Geometry: final body of the model. Coordinates: model frame, mm. Face numbers are marked on the shaded views. A direction names the side the tool comes from. Give positions to 0.01 mm unless a question says otherwise; leave off trailing zeros. Write each loop counter-clockwise with the first axis right and the second up, starting at its lowest first coordinate (ties: lowest second). Pieces come first, ordered by that corner, then holes.
from build123d import *

# Parameters (mm, degrees)
SKETCH1_W              = 70
SKETCH1_H              = 20
BASE_FLANGE1_DEPTH     = 3
SKETCHED_BEND1_DEPTH   = 20
SKETCHED_BEND1_2_DEPTH = 20
FILLET1_R              = 10
SKETCH10_R             = 4.5
CUT_EXTRUDE1_DEPTH     = 46.126468159


# Read off the part's stored shape, not the designer's step: Sketched Bend1
# Sheet-metal steps are written as plain solids
with BuildPart() as part:
    # Sketch1 → Base-Flange1 (new body)
    with BuildSketch(Plane.XY):
        with Locations((35, 10)):
            Rectangle(SKETCH1_W, SKETCH1_H)
    extrude(amount=-BASE_FLANGE1_DEPTH)

    # Sketched Bend1 outline → Sketched Bend1 (cut)
    with BuildSketch(Plane(origin=(0, 0, 0), x_dir=(1, 0, 0), z_dir=(0, 1, 0))):
        with BuildLine():
            ThreePointArc((18.243378468, 3), (20.610845469, 2.154295979), (21.906655689, 0))
            Line((21.906655689, 0), (70, 0))
            Line((70, 0), (70, 3))
            Line((70, 3), (18.243378468, 3))
        make_face()
    extrude(amount=SKETCHED_BEND1_DEPTH, mode=Mode.SUBTRACT)

    # Sketched Bend1 2 outline → Sketched Bend1 2 (add)
    with BuildSketch(Plane(origin=(0, 0, 0), x_dir=(1, 0, 0), z_dir=(0, 1, 0))):
        with BuildLine():
            Line((18.979978468, -0.7366), (18.979978468, -27.223356935))
            ThreePointArc((18.979978468, -27.223356935), (18.764233323, -27.74421179), (18.243378468, -27.959956935))
            Line((18.243378468, -27.959956935), (0, -27.959956935))
            Line((0, -27.959956935), (0, -30.959956935))
            Line((0, -30.959956935), (18.243378468, -30.959956935))
            ThreePointArc((18.243378468, -30.959956935), (20.885553666, -29.865532134), (21.979978468, -27.223356935))
            Line((21.979978468, -27.223356935), (21.979978468, -0.7366))
            ThreePointArc((21.979978468, -0.7366), (21.961602589, -0.36647982), (21.906655689, 0))
            Line((21.906655689, 0), (18.243378468, 0))
            ThreePointArc((18.243378468, 0), (18.764233323, -0.215745145), (18.979978468, -0.7366))
        make_face()
    extrude(amount=SKETCHED_BEND1_2_DEPTH)

    # Fillet1
    fillet1_edges = [part.edges().sort_by_distance(p)[0] for p in [
        (0, 0, 29.459956935),
        (0, 0, -1.5),
        (0, 20, 29.459956935),
        (0, 20, -1.5),
    ]]
    fillet(fillet1_edges, radius=FILLET1_R - 0.0001)  # a hair under: the kernel refuses the full size

    # Sketch10 → Cut-Extrude1 (cut, through all)
    with BuildSketch(Plane.XY.offset(30.959956935)):
        with Locations((10, 10)):
            Circle(SKETCH10_R)
    extrude(amount=-CUT_EXTRUDE1_DEPTH, mode=Mode.SUBTRACT)


solid = part.part
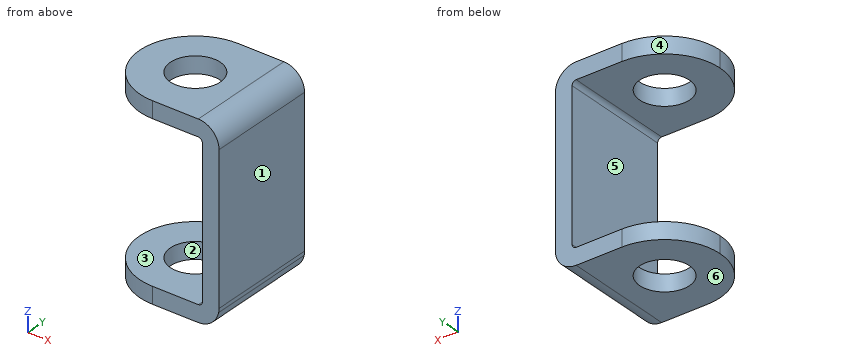
Q1. Section D-D on y = 16.5. Output: boundary loops of the cut face in (x, z), plus the area to 3 significant figures.
Filled sheet:
outline: (2.4, -3) - (18.24, -3) arc R3.74 ccw to (21.98, 0.74) - (21.98, 27.22) arc R3.74 ccw to (18.24, 30.96) - (2.4, 30.96) - (2.4, 27.96) - (18.24, 27.96) arc R0.74 cw to (18.98, 27.22) - (18.98, 0.74) arc R0.74 cw to (18.24, 0) - (2.4, 0) - close
area: 196 mm2
Q2. Pull-direction query (X, two-part tool) for the marked faces 1, 2, 3 and 4; classes: released by +X, released by -X, zero draft, split by the parting line, or undercut.
Filled sheet:
face 1: released by +X
face 2: undercut
face 3: zero draft
face 4: released by -X
Q3. Section C-C on y = 8.75. Output: boundary loops of the cut face in (x, z).
Filled sheet:
outline: (0.08, -3) - (5.68, -3) - (5.68, 0) - (0.08, 0) - close; (0.08, 27.96) - (5.68, 27.96) - (5.68, 30.96) - (0.08, 30.96) - close; (14.32, -3) - (18.24, -3) arc R3.74 ccw to (21.98, 0.74) - (21.98, 27.22) arc R3.74 ccw to (18.24, 30.96) - (14.32, 30.96) - (14.32, 27.96) - (18.24, 27.96) arc R0.74 cw to (18.98, 27.22) - (18.98, 0.74) arc R0.74 cw to (18.24, 0) - (14.32, 0) - close
Q4. Access query for the marked faces 5 and 6. Directions: +Z, -Z, +X, -X, +Y, -Y. A direction counts if a zero-diameter tool reaches every point of the face in a straight line with its end or side. Return the directions, or none.
Filled sheet:
face 5: -X, +Y, -Y
face 6: -Z, +X, -X, +Y, -Y
Q5. Ray query, line 1 along Z through (x, y) = (8, 14.5); line 2 along Y through (x, z) = (10, -2.1); line 3 along X through (y, z) = (4, 6). Return the intervals inside material, ascending.
Filled sheet:
line 1: z = -3 to 0, 27.96 to 30.96
line 2: y = 0 to 5.5, 14.5 to 20
line 3: x = 18.98 to 21.98
Q6. Pin query (flat end, axial travel): P1, Ø5, axis at y = 15.5, z = 24.5, coming from the -X side. Return the tip coordinate at first contact, or that it passes through.
Filled sheet:
P1: stops at x = 18.98
Q7. Section B-B on x = 8.5. Output: boundary loops of the cut face in (y, z).
Filled sheet:
outline: (0.11, -3) - (5.76, -3) - (5.76, 0) - (0.11, 0) - close; (0.11, 27.96) - (5.76, 27.96) - (5.76, 30.96) - (0.11, 30.96) - close; (14.24, -3) - (19.89, -3) - (19.89, 0) - (14.24, 0) - close; (14.24, 27.96) - (19.89, 27.96) - (19.89, 30.96) - (14.24, 30.96) - close
Q8. Section A-A on x = 17.5. Output: boundary loops of the cut face in (y, z), plus the area to 3 significant figures.
Filled sheet:
outline: (0, -3) - (20, -3) - (20, 0) - (0, 0) - close; (0, 27.96) - (20, 27.96) - (20, 30.96) - (0, 30.96) - close
area: 120 mm2
